from build123d import *

# Parameters (mm, degrees)
SKETCH10_R          = 1.5875
BOSS_EXTRUDE2_DEPTH = 5.55625
CUT_EXTRUDE5_DEPTH  = 2.38125
CUT_EXTRUDE6_DEPTH  = 2.38125
FILLET2_R           = 0.79375
CHAMFER2_SIZE       = 0.508


with BuildPart() as part:
    # Sketch10 → Boss-Extrude2 (new body)
    with BuildSketch(Plane.XY):
        with BuildLine():
            Line((-12.489905714, 4.426128528), (-2.358571429, 7.578987206))
            ThreePointArc((-2.358571429, 7.578987206), (0, 7.9375), (2.358571429, 7.578987206))
            Line((2.358571429, 7.578987206), (12.489905714, 4.426128528))
            ThreePointArc((12.489905714, 4.426128528), (15.748, 0), (12.489905714, -4.426128528))
            Line((12.489905714, -4.426128528), (2.358571429, -7.578987206))
            ThreePointArc((2.358571429, -7.578987206), (0, -7.9375), (-2.358571429, -7.578987206))
            Line((-2.358571429, -7.578987206), (-12.489905714, -4.426128528))
            ThreePointArc((-12.489905714, -4.426128528), (-15.748, 0), (-12.489905714, 4.426128528))
        make_face()
        Circle(SKETCH10_R, mode=Mode.SUBTRACT)
        with Locations((-11.1125, 0)):
            Circle(SKETCH10_R, mode=Mode.SUBTRACT)
        with Locations((11.1125, 0)):
            Circle(SKETCH10_R, mode=Mode.SUBTRACT)
    extrude(amount=BOSS_EXTRUDE2_DEPTH)

    # Sketch11 → Cut-Extrude5 (cut)
    with BuildSketch(Plane.XY.offset(5.55625)):
        Polygon((-11.1125, 3.519527241), (-14.1605, 1.75976362), (-14.1605, -1.75976362), (-11.1125, -3.519527241), (-8.0645, -1.75976362), (-8.0645, 1.75976362), align=None)
        Polygon((14.1605, 1.75976362), (11.1125, 3.519527241), (8.0645, 1.75976362), (8.0645, -1.75976362), (11.1125, -3.519527241), (14.1605, -1.75976362), align=None)
    extrude(amount=-CUT_EXTRUDE5_DEPTH, mode=Mode.SUBTRACT)

    # Sketch12 → Cut-Extrude6 (cut)
    with BuildSketch(Plane(origin=(0, 0, 0), x_dir=(-1, 0, 0), z_dir=(0, 0, -1))):
        Polygon((3.048, 1.75976362), (0, 3.519527241), (-3.048, 1.75976362), (-3.048, -1.75976362), (0, -3.519527241), (3.048, -1.75976362), align=None)
    extrude(amount=-CUT_EXTRUDE6_DEPTH, mode=Mode.SUBTRACT)

    # Fillet2
    fillet2_edges = [part.edges().sort_by_distance(p)[0] for p in [
        (-9.5885, 2.639645431, 3.175),
        (-11.1125, 3.519527241, 4.365625),
        (-8.0645, 0, 3.175),
        (-8.0645, 1.75976362, 4.365625),
        (-9.5885, -2.639645431, 3.175),
        (-8.0645, -1.75976362, 4.365625),
        (-12.6365, -2.639645431, 3.175),
        (-11.1125, -3.519527241, 4.365625),
        (-14.1605, 0, 3.175),
        (-14.1605, -1.75976362, 4.365625),
        (-12.6365, 2.639645431, 3.175),
        (-14.1605, 1.75976362, 4.365625),
        (14.1605, 0, 3.175),
        (14.1605, 1.75976362, 4.365625),
        (12.6365, -2.639645431, 3.175),
        (14.1605, -1.75976362, 4.365625),
        (9.5885, -2.639645431, 3.175),
        (11.1125, -3.519527241, 4.365625),
        (8.0645, 0, 3.175),
        (8.0645, -1.75976362, 4.365625),
        (9.5885, 2.639645431, 3.175),
        (8.0645, 1.75976362, 4.365625),
        (12.6365, 2.639645431, 3.175),
        (11.1125, 3.519527241, 4.365625),
        (-3.048, 0, 2.38125),
        (-3.048, 1.75976362, 1.190625),
        (-1.524, -2.639645431, 2.38125),
        (-3.048, -1.75976362, 1.190625),
        (1.524, -2.639645431, 2.38125),
        (0, -3.519527241, 1.190625),
        (3.048, 0, 2.38125),
        (3.048, -1.75976362, 1.190625),
        (1.524, 2.639645431, 2.38125),
        (3.048, 1.75976362, 1.190625),
        (-1.524, 2.639645431, 2.38125),
        (0, 3.519527241, 1.190625),
    ]]
    fillet(fillet2_edges, radius=FILLET2_R)

    # Chamfer2
    chamfer2_edges = [part.edges().sort_by_distance(p)[0] for p in [
        (7.424238571, -6.002557867, 0),
        (0, -7.9375, 0),
        (-1.524, 2.639645431, 0),
        (1.524, 2.639645431, 0),
        (-7.424238571, -6.002557867, 0),
        (3.048, 0, 0),
        (1.524, -2.639645431, 0),
        (-15.748, 0, 0),
        (-1.524, -2.639645431, 0),
        (-3.048, 0, 0),
        (14.1605, 0, 5.55625),
        (12.6365, 2.639645431, 5.55625),
        (9.5885, 2.639645431, 5.55625),
        (8.0645, 0, 5.55625),
        (0, -7.9375, 5.55625),
        (9.5885, -2.639645431, 5.55625),
        (12.6365, -2.639645431, 5.55625),
        (-9.5885, 2.639645431, 5.55625),
        (-12.6365, 2.639645431, 5.55625),
        (-14.1605, 0, 5.55625),
        (-12.6365, -2.639645431, 5.55625),
        (-9.5885, -2.639645431, 5.55625),
        (-8.0645, 0, 5.55625),
        (-2.941657664, 1.698366844, 0),
        (0, 3.396733689, 0),
        (2.941657664, 1.698366844, 0),
        (2.941657664, -1.698366844, 0),
        (0, -3.396733689, 0),
        (-2.941657664, -1.698366844, 0),
        (14.054157664, 1.698366844, 5.55625),
        (11.1125, 3.396733689, 5.55625),
        (8.170842336, 1.698366844, 5.55625),
        (8.170842336, -1.698366844, 5.55625),
        (11.1125, -3.396733689, 5.55625),
        (14.054157664, -1.698366844, 5.55625),
        (-11.1125, 3.396733689, 5.55625),
        (-14.054157664, 1.698366844, 5.55625),
        (-11.1125, -3.396733689, 5.55625),
        (-8.170842336, -1.698366844, 5.55625),
        (-8.170842336, 1.698366844, 5.55625),
        (-14.054157664, -1.698366844, 5.55625),
        (7.424238571, -6.002557867, 5.55625),
        (15.748, 0, 5.55625),
        (-1.5875, 0, 5.55625),
        (7.424238571, 6.002557867, 5.55625),
        (-12.7, 0, 0),
        (0, 7.9375, 5.55625),
        (9.525, 0, 0),
        (-7.424238571, 6.002557867, 5.55625),
        (-12.7, 0, 3.175),
        (-15.748, 0, 5.55625),
        (9.525, 0, 3.175),
        (-1.5875, 0, 2.38125),
        (-7.424238571, 6.002557867, 0),
        (-7.424238571, -6.002557867, 5.55625),
        (0, 7.9375, 0),
        (7.424238571, 6.002557867, 0),
        (15.748, 0, 0),
    ]]
    chamfer(chamfer2_edges, length=CHAMFER2_SIZE)


solid = part.part
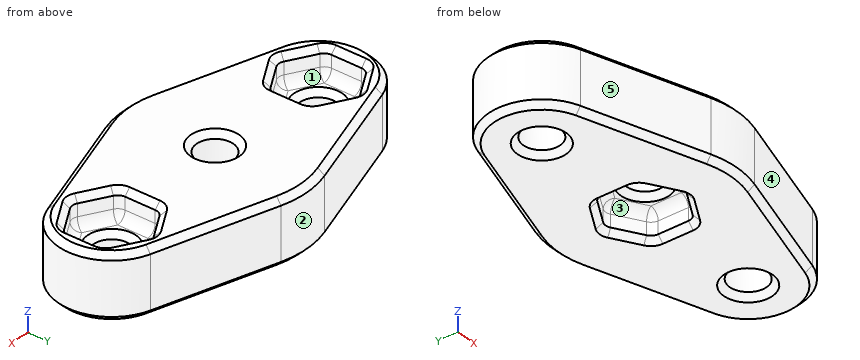
Read the model definition and answer for the solid it produces. Units are mm, in the model's axes. Face numbers are marked on the shaded views. A direction names the side the tool comes from. Coordinates: 2 decimals unless noted, no trailing zeros. Write each loop counter-clockwise with the first axis right and the second up, starting at its lowest first coordinate (ties: lowest second). Pieces come first, ordered by that corner, then holes. Notation, with made-up numbers: (11.25, -38.5) - (43.25, -38.5) arc R18 ccw to (43.25, -17.5) - close; hole circle Ø10 at (-31.5, 7.5). An arc over 180 degrees is marked (long way). One line per question, with ' | ' between items.
Q1. Determine the mould class of the marked faces 3, 4 and 5 for opening direction X: +X half, -X half, draft (parallel to the pull), parting line (faces both ways), or undercut.
Result set:
face 3: undercut | face 4: +X half | face 5: -X half
Q2. Find section C-C, the plane x = -7. Write down the section's boundary in (y, z), plus the area to 3 significant figures.
Result set:
outline: (-6.13, 0.51) - (-5.6, 0) - (5.6, 0) - (6.13, 0.51) - (6.13, 5.05) - (5.6, 5.56) - (-5.6, 5.56) - (-6.13, 5.05) - close | area: 67.6 mm^2
Q3. Find section D-D, the plane y = 6.5. Write down the section's boundary in (x, z).
Result set:
outline: (-5.83, 0.51) - (-4.12, 0) - (4.12, 0) - (5.83, 0.51) - (5.83, 5.05) - (4.12, 5.56) - (-4.12, 5.56) - (-5.83, 5.05) - close
Q4. Each of these flat-tipped pins is pushed along its axis until it touches: P1, Ø1, axis at y = 3, z = 2.5, coming from the -X side; P2, Ø3.5, axis at x = -10.5, y = 0.5, coming from the +Z side; P3, Ø3.5, axis at x = 0.5, y = 0, coming from the -Z side. Where does it stop, or does it pass through?
Result set:
P1: x = -15.02 | P2: z = 3.21 | P3: z = 2.38
Q5. For the marked faces 1 and 2, determine the directions among +Z, -Z, +X, -X, +Y, -Y from which every point of the face is accessible in a straight line to the end or side of a thin tool.
Result set:
face 1: +Z | face 2: +Z, -Z, +Y
Q6. Find section A-A, the plane z = 4.45. State how many separate pieces and enclosed holes the cut face has, plus the area to 3 significant figures.
Result set:
separate pieces: 1 | enclosed holes: 3 | area: 287 mm^2
Q7. Consider L1, parallel to X at y = 0, z = 1.25 (3 decimals); L2, parallel to Y at x = 0, z = 4.1; L3, parallel to Z at x = -2, y = 1. Determine where each line is inside the solid, lowest interval first. Write a range as [from, to].
Result set:
L1: [-15.748, -12.7], [-9.525, -3.048], [3.048, 9.525], [12.7, 15.748] | L2: [-7.94, -1.59], [1.59, 7.94] | L3: [2.38, 5.56]
